Geometry check sheet. Reference: the model listing, model coordinates, mm. A direction names the side the tool comes from. Coordinates: 2 decimals unless noted, no trailing zeros. Order: outer loops, then holes, each group sorted by start corner. A loop starts at its lowest first (then second) coordinate and runs counter-clockwise, first axis right, second up. Notation, with made-up numbers: (17, -35) - (42, -35) arc R30 ccw to (42, -5) - close; hole circle Ø11 at (-4, 52). An arc over 180 degrees is marked (long way). Put each result on its own line as item: value.
Autodesk Inventor part; units mm, degrees
ref_plane "YZ Plane" through (0, 0, 0) normal (1, 0, 0) x (0, 1, 0)
ref_plane "XZ Plane" through (0, 0, 0) normal (0, 1, 0) x (-1, 0, 0)
ref_plane "XY Plane" through (0, 0, 0) normal (0, 0, 1) x (1, 0, 0)
sketch "Sketch1" plane through (0, 0, 0) normal (1, 0, 0) x (0, 1, 0)
  circle A0 centre (0, 0) radius 6.477
  circle A1 centre (0, 0) radius 12.827
  dimension "d0" = 12.954
  dimension "d1" = 25.654
extrude "Extrusion1" add sketch "Sketch1" along normal blind 50.8
sketch "Sketch2" plane through (50.8, 0, 0) normal (1, 0, 0) x (0, 0, -1)
  circle A0 centre (0, 0) radius 12.827
  circle A1 centre (0, 0) radius 6.477
  line L0 (0, 0) -> (0, 12.827) construction
  line L1 (0, 12.827) -> (-3.81, 12.827)
  arc A2 (-12.827, 0) -> (12.827, 0) centre (0, 0) ccw construction
  line L2 (0, 0) -> (12.827, 0) construction
  line L3 (0, 0) -> (-12.827, 0) construction
  line L4 (-12.827, 0) -> (-12.827, 12.827)
  line L5 (-12.827, 12.827) -> (0, 12.827)
  line L6 (12.827, 12.827) -> (12.827, 0)
  circle A3 centre (0, 0) radius 12.827
  line L7 (12.827, 12.827) -> (3.81, 12.827) construction
  arc A4 (0, 12.827) -> (-12.827, 0) centre (0, 0) ccw
  arc A5 (12.827, 0) -> (0, 12.827) centre (0, 0) ccw
  line L8 (0, 12.827) -> (3.81, 12.827)
  line L9 (3.81, 12.827) -> (3.81, 22.987)
  line L10 (3.81, 22.987) -> (12.827, 22.987)
  line L11 (12.827, 22.987) -> (12.827, 12.827)
  line L12 (3.81, 12.827) -> (0, 12.827)
  point P0 (12.827, 0)
  dimension "d5" = 3.81
  dimension "d6" = 10.16
extrude "Extrusion2" add sketch "Sketch2" against normal blind 50.8 contours A0 L8 L9 L10 L11 L6 | A0 L4 L5 L1
sketch "Sketch3" plane through (50.8, 12.827, -3.81) normal (0, 0, 1) x (1, 0, 0)
  line L0 (0, 0) -> (-50.8, 0)
  line L1 (0, 10.16) -> (-50.8, 10.16)
  line L2 (-50.8, 0) -> (-50.8, 10.16)
  line L3 (0, 10.16) -> (0, 0)
  line L4 (-25.4, 10.16) -> (-25.4, 0) construction
  line L5 (-25.4, 5.08) -> (-17.78, 5.08) construction
  circle A0 centre (-17.78, 5.08) radius 2.413
  circle A1 centre (-33.02, 5.08) radius 2.413
  point P0 (-50.8, -12.827)
  dimension "d9" = 7.62
  dimension "d11" = 4.826
extrude "Extrusion3" cut sketch "Sketch3" against normal through all contours A0 | A1
sketch "Sketch4" plane through (50.8, 12.827, 12.827) normal (0, 1, 0) x (1, 0, 0)
  line L0 (0, 16.637) -> (0, 0)
  line L1 (0, 16.637) -> (-50.8, 16.637)
  line L2 (-50.8, 0) -> (-50.8, 16.637)
  line L3 (0, 0) -> (-50.8, 0)
  line L4 (-25.4, 0) -> (-25.4, 16.637) construction
  line L5 (0, 19.304) -> (0, 6.35)
  line L6 (0, 12.827) -> (-50.8, 12.827) construction
  circle A0 centre (-25.4, 12.827) radius 2.413
  dimension "d15" = 4.826
extrude "Extrusion4" cut sketch "Sketch4" against normal through all contours A0
properties part number "arm_to_camera"
Q1. Depth check by flat-ended pin: pin 1 Ø1.5 at (x, z) = (16.5, -0.5) entering from +Y; pin 2 Ø4.5 at (x, y) = (33.02, 17.907) entering from +Z; pin 3 Ø6 at (x, y) = (45, -8.5) entering from +Z; pin 4 Ø1 at (x, z) = (13, -1.5) entering from -Y. Enter the tip coordinate at first touch or a pass-through.
Answer block:
pin 1: stops at y = 12.83
pin 2: passes through
pin 3: stops at z = 11.59
pin 4: stops at y = -12.79
Q2. Access from +Z, -Z, +X, -X, +Y, -Y to the whole of each face (thin tool, end or side, straight path). Record for faces 1 (the flat face through (26, 18, -3.81)), 2 (the flat face through (26, 12, -12.827)).
Answer block:
face 1: +Z, +X, -X, +Y
face 2: -Z, +X, -X, +Y, -Y
Q3. Section check B-B on z = 0. Record the boundary of the cut face in (x, y), then the cut area to 3 significant figures.
Answer block:
outline: (0, -12.83) - (22.99, -12.83) - (22.99, -6.48) - (0, -6.48) - close; (0, 6.48) - (22.99, 6.48) - (22.99, 12.83) - (0, 12.83) - close; (27.81, -12.83) - (50.8, -12.83) - (50.8, -6.48) - (27.81, -6.48) - close; (27.81, 6.48) - (50.8, 6.48) - (50.8, 12.83) - (27.81, 12.83) - close
area: 584 mm^2
Q4. Section check D-D on x = 8. Record the boundary of the cut face in (y, z).
Answer block:
outline: (0, -12.83) - (22.99, -12.83) - (22.99, -3.81) - (12.83, -3.81) - (12.83, 12.83) - (0, 12.83) arc R12.83 ccw to start; hole circle Ø12.95 at (0, 0)
Q5. Section check A-A on x = 33.02. Record the boundary of the cut face in (y, z).
Answer block:
outline: (0, -12.83) - (15.49, -12.83) - (15.49, -3.81) - (12.83, -3.81) - (12.83, 12.83) - (0, 12.83) arc R12.83 ccw to start; (20.32, -12.83) - (22.99, -12.83) - (22.99, -3.81) - (20.32, -3.81) - close; hole circle Ø12.95 at (0, 0)
Q6. Section check C-C on y = 19.5. Record the boundary of the cut face in (x, z).
Answer block:
outline: (0, -12.83) - (15.97, -12.83) - (15.97, -3.81) - (0, -3.81) - close; (19.59, -12.83) - (31.21, -12.83) - (31.21, -3.81) - (19.59, -3.81) - close; (34.83, -12.83) - (50.8, -12.83) - (50.8, -3.81) - (34.83, -3.81) - close
Q7. Draft check along X on faces 3 (the flat face through (0, 9, 0)), 4 (the cylindrical face through (27.63, 9.47, 0.92)), 5 (the flat face through (26, 22.987, -8)). Enter one of: pulls with the +X half, pulls with the -X half, needs draft (parallel to the pull), parting line crosses it, or undercut.
Answer block:
face 3: pulls with the -X half
face 4: undercut
face 5: needs draft
Q8. Thickness scan on L1, parallel to Z at x = 20, y = 0; L2, parallel to Z at x = 25.4, y = 8; L3, parallel to X at y = -8, z = 0. Record the ranges inside material, lowest first. Write a range as [from, to].
Answer block:
L1: z = [-12.83, -6.48], [6.48, 12.83]
L2: z = [-12.83, -2.41], [2.41, 12.83]
L3: x = [0, 22.99], [27.81, 50.8]
